Check sheet for the modelled part. Datum: model origin and axes. Units: mm. Face numbers are marked on the shaded views. A direction names the side the tool comes from. Round coordinates to 2 decimals unless told otherwise and drop trailing zeros. Write each loop counter-clockwise with the first axis right and the second up, starting at its lowest first coordinate (ties: lowest second). Pieces come first, ordered by that corner, then holes. Notation, with made-up numbers: (40.5, -31.75) -> (87.5, -31.75) arc R22 cw to (87.5, -4.75) -> close; hole circle Ø5 at (53, 6). An arc over 180 degrees is marked (long way). One line per item, written item: value. Start each with the question number.
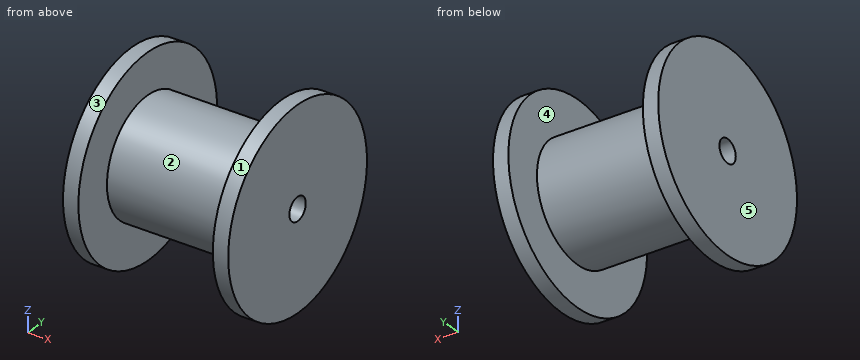
```python
from build123d import *

# Parameters (mm, degrees)
SKETCH8_R          = 3
CUT_EXTRUDE1_DEPTH = 57.120406271


with BuildPart() as part:
    # Sketch1 → Revolve1 (revolve)
    with BuildSketch(Plane.XY, mode=Mode.PRIVATE) as revolve1_sk:
        Polygon((0, 0), (0, 3), (0, 25.5), (4, 25.5), (4, 15), (39, 15), (39, 25.5), (43, 25.5), (43, 3), (43, 0), align=None)
    revolve(revolve1_sk.sketch.rotate(Axis((0, 0, 0), (1, 0, 0)), 90), axis=Axis((0, 0, 0), (1, 0, 0)))

    # Sketch8 → Cut-Extrude1 (cut, through all)
    with BuildSketch(Plane.ZY):
        Circle(SKETCH8_R)
    extrude(amount=-CUT_EXTRUDE1_DEPTH, mode=Mode.SUBTRACT)


solid = part.part
```
1. Material ranges on probe 1 along X at (y, z) = (13, -15.5); probe 2 along Y at (x, z) = (30, 0); probe 3 along Z at (x, y) = (14, -11), recorded low to high.
2. Cross-section at A-A (y = 0). Record the cut outline in (x, z), plus the area to 3 significant figures.
3. Cross-section at C-C (z = 12). Record the cut outline in (x, y), plus the area to 3 significant figures.
4. Release check for a two-part mould opening along X. For the marked faces 3, 4 and 5 record: +X half, -X half, draft (parallel to the pull), parting line (faces both ways), or undercut.
5. Access from +Z, -Z, +X, -X, +Y, -Y to the whole of each face (thin tool, end or side, straight path). Record for the marked faces 1 and 2.
6. Cross-section at D-D (x = 7). Record the cut outline in (y, z).
7. Depth check by flat-ended pin: pin 1 Ø1 at (x, y) = (7, 7.5) entering from +Z; pin 2 Ø2 at (x, y) = (28.5, 2.5) entering from +Z; pin 3 Ø4 at (y, z) = (11, -5) entering from -X; pin 4 Ø6 at (x, z) = (23, 7) entering from +Y. Enter the tip coordinate at first touch or a pass-through.
Working result:
1. probe 1: x = 0 to 4, 39 to 43
1. probe 2: y = -15 to -3, 3 to 15
1. probe 3: z = -10.2 to 10.2
2. outline: (0, -25.5) -> (4, -25.5) -> (4, -15) -> (39, -15) -> (39, -25.5) -> (43, -25.5) -> (43, -3) -> (0, -3) -> close; (0, 3) -> (43, 3) -> (43, 25.5) -> (39, 25.5) -> (39, 15) -> (4, 15) -> (4, 25.5) -> (0, 25.5) -> close
2. area: 1,200 mm^2
3. outline: (0, -22.5) -> (4, -22.5) -> (4, -9) -> (39, -9) -> (39, -22.5) -> (43, -22.5) -> (43, 22.5) -> (39, 22.5) -> (39, 9) -> (4, 9) -> (4, 22.5) -> (0, 22.5) -> close
3. area: 990 mm^2
4. face 3: draft
4. face 4: undercut
4. face 5: -X half
5. face 1: +X, -X
5. face 2: none
6. outline: circle Ø30 at (0, 0); hole circle Ø6 at (0, 0)
7. pin 1: stops at z = 13.27
7. pin 2: stops at z = 14.92
7. pin 3: stops at x = 0
7. pin 4: stops at y = 14.46
